For this review, use the dimensioned drawing (mm, ordinates from the lowest corner) and the shaded views. Give positions to 0.01 mm unless a question says otherwise; leave off trailing zeros. Order: outer loops, then holes, each group sorted by start corner. A loop starts at its lowest first (then second) coordinate and runs counter-clockwise, first axis right, second up. Notation, with made-up numbers: (29, -29) - (44, -29) arc R21 cw to (44, -17) - close; hole circle Ø7 at (31.25, 50). An arc over 180 degrees is marked (long way). Use a Markdown table: item, result. Add a question column.
1) We need section A-A on z = 198. Write out the cut boundary in (x, y).
2) Clearance check with flat-ended pins moving along their axes: P1, Ø2, axis at y = 51, z = 165.5, coming from the -X side; P2, Ø3, axis at x = 41.5, z = 226.5, coming from the +Y side; P3, Ø12, axis at y = 11, z = 330, coming from the +X side. State where each tip first meets the part, or that it passes through.
3) Wall thickness on L1, parallel to Y at x = 20.5, z = 64.5; L2, parallel to Y at x = 30.5, z = 30.5; L3, parallel to X at y = 24.5, z = 265: over which ranges is each line inside the solid? List them lowest first.
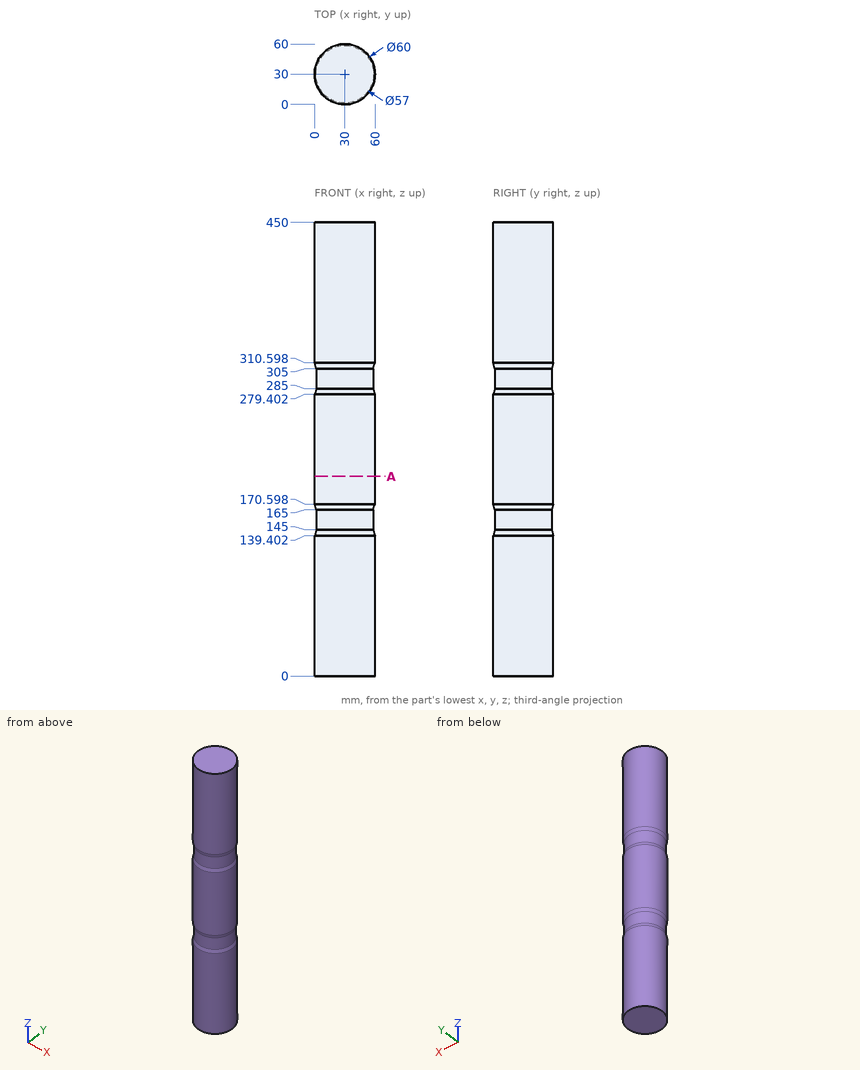
Checked values:
| question | item | result |
|---|---|---|
| 1 | outline | circle Ø60 at (30, 30) |
| 2 | P1 | x = 9.44 |
| 2 | P2 | y = 58.28 |
| 2 | P3 | x = 57.04 |
| 3 | L1 | 1.54 to 58.46 |
| 3 | L2 | 0 to 60 |
| 3 | L3 | 0.51 to 59.49 |
